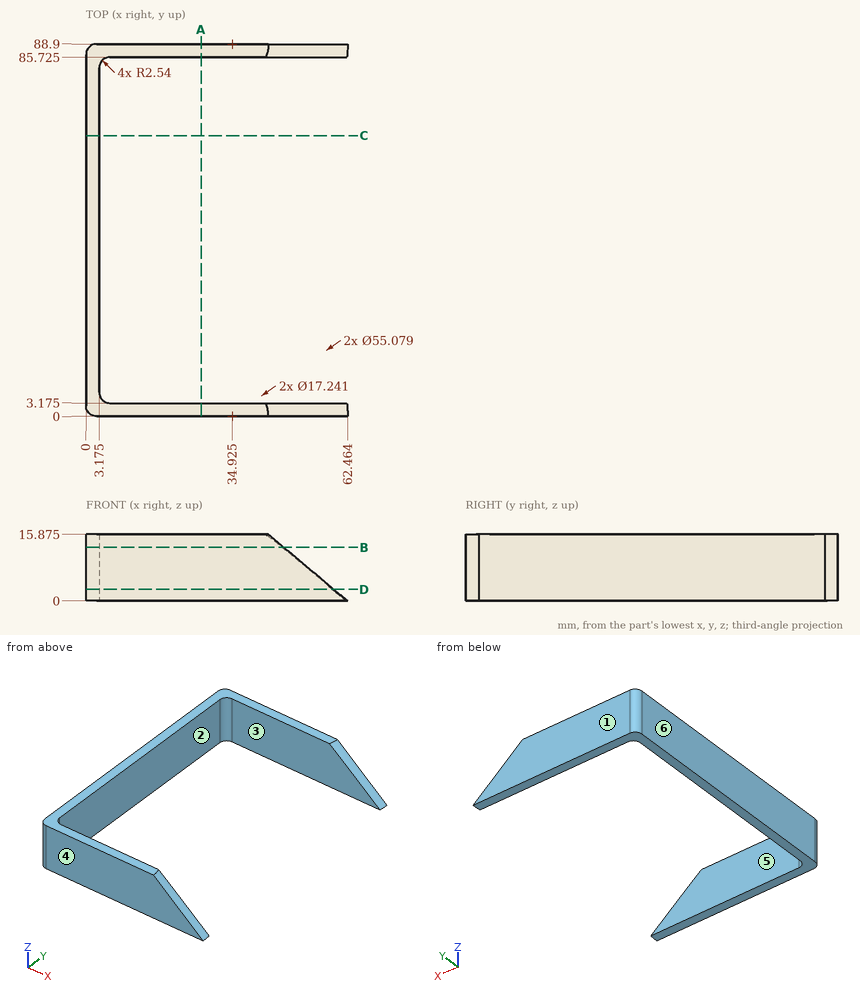
Design review of the part shown in the three views and the two pictorial views. Dimensions are in mm from the part's minimum x, y and z. A direction names the side the tool comes from. Round coordinates to 2 decimals unless told otherwise and drop trailing zeros. Loops run counter-clockwise (first coordinate to the right, second up) from the corner with the lowest first, then second, coordinate; pieces in that order, holes last. Notation, with made-up numbers: M 79.25,24.25 L 109.25,24.25 A15 ccw 109.25,48.25 Z; hole C -8,-23.75 d4. An arc over 180 degrees is marked long. Write item = value, one per line.
Item 1: Machinability: for the marked faces 5 and 6, which of the approach directions +Z, -Z, +X, -X, +Y, -Y give a long, thin tool a straight path to every point of the face, cutting with its end or side? Answer none if there is none.
Return value:
face_5 = +Z, -Z, +X
face_6 = +Z, -Z, -X, +Y, -Y
Item 2: The part is to be moulded in two halves that separate along Y. For the marked faces 1, 2, 3 and 4, say which applies: released by +Y, released by -Y, zero draft, split by the parting line, or undercut.
Return value:
face_1 = released by +Y
face_2 = undercut
face_3 = undercut
face_4 = released by -Y
Item 3: Insertion check: P1, Ø1.5, axis at y = 43, z = 14, coming from the +X side (3 decimals). The pin has a flat end and moves straight along its axis. Give the tip position at first contact, or say it passes through.
Return value:
P1 = 3.175
Item 4: Take a section at A-A on x = 27.5. Write out the cut boundary in (y, z) (1 decimal).
Return value:
outline = M 0,0 L 3.2,0 L 3.2,15.9 L 0,15.9 Z; M 85.7,0 L 88.9,0 L 88.9,15.9 L 85.7,15.9 Z
Item 5: Take a section at D-D on z = 2.75. Write out the cut boundary in (x, y) (1 decimal).
Return value:
outline = M 0,2.5 A2.5 ccw 2.5,0 L 59.2,0 A24.3 ccw 59,3.2 L 5.7,3.2 A2.5 cw 3.2,5.7 L 3.2,83.2 A2.5 cw 5.7,85.7 L 59,85.7 A24.3 ccw 59.2,88.9 L 2.5,88.9 A2.5 ccw 0,86.4 Z
Item 6: Take a section at B-B on z = 12.75. Write out the cut boundary in (x, y) (1 decimal).
Return value:
outline = M 0,2.5 A2.5 ccw 2.5,0 L 47.3,0 A12.3 ccw 46.9,3.2 L 5.7,3.2 A2.5 cw 3.2,5.7 L 3.2,83.2 A2.5 cw 5.7,85.7 L 46.9,85.7 A12.3 ccw 47.3,88.9 L 2.5,88.9 A2.5 ccw 0,86.4 Z
Item 7: For line 1 (Y direction, x = 23.5, z = 5.75) (1 decimal); line 2 (X direction, y = 82.5, z = 4.75) (1 decimal); line 3 (Y direction, x = 5, z = 8.75), list the stretches that pass through material, from the lowest coordinate up. Write a range as [from, to].
Return value:
line_1 = [0, 3.2], [85.7, 88.9]
line_2 = [0, 3.2]
line_3 = [0, 3.28], [85.62, 88.9]
Item 8: Take a section at C-C on y = 67. Write out the cut boundary in (x, z) (1 decimal).
Return value:
outline = M 0,0 L 3.2,0 L 3.2,15.9 L 0,15.9 Z
